Verification items for the finished model (mm, model axes). A direction names the side the tool comes from. Round coordinates to 2 decimals unless told otherwise and drop trailing zeros. Loops run counter-clockwise (first coordinate to the right, second up) from the corner with the lowest first, then second, coordinate; pieces in that order, holes last. Notation, with made-up numbers: (0.5, 0.5) - (30.5, 0.5) arc R21 cw to (30.5, 6.5) - close; hole circle Ø11 at (63, 69). An arc over 180 degrees is marked (long way). Use CSV: the item, a comma, the result in double quotes.
Autodesk Inventor part; units mm, degrees
ref_plane "YZ Plane" through (0, 0, 0) normal (1, 0, 0) x (0, 1, 0)
ref_plane "XZ Plane" through (0, 0, 0) normal (0, 1, 0) x (-1, 0, 0)
ref_plane "XY Plane" through (0, 0, 0) normal (0, 0, 1) x (1, 0, 0)
sketch "Sketch1" plane through (0, 0, 0) normal (0, 0, 1) x (1, 0, 0)
  line L0 (-35, 0) -> (0, 0)
  line L1 (0, 0) -> (0, 10)
  line L2 (0, 10) -> (-35, 10)
  line L3 (-35, 10) -> (-35, 0)
  dimension "d0" = 35
  dimension "d1" = 10
extrude "Extrusion1" add sketch "Sketch1" along normal blind 30
sketch "Sketch2" plane through (-35, 10, 0) normal (0, 1, 0) x (1, 0, 0)
  line L0 (35, -30) -> (0, -30) construction
  line L1 (17.5, -30) -> (17.5, 0) construction
  line L2 (0, 0) -> (35, 0) construction
  circle A0 centre (17.5, -15) radius 11.25
  point P0 (30, -30)
  point P1 (5, -30)
  point P2 (5, 0)
  point P3 (30, 0)
  dimension "d5" = 22.5
extrude "Extrusion2" cut sketch "Sketch2" against normal blind 7.5
sketch "Sketch3" plane through (0, 0, 0) normal (0, 0, -1) x (-1, 0, 0)
  line L0 (0, 10) -> (35, 10) construction
  line L1 (17.5, 10) -> (17.5, 0) construction
  line L2 (30, 0) -> (5, 0) construction
  circle A0 centre (4, 5) radius 1.65
  circle A1 centre (31, 5) radius 1.65
  line L3 (0, 0) -> (0, 10)
  line L4 (35, 10) -> (35, 0)
  point P0 (5, 10)
  point P1 (30, 10)
  point P2 (17.5, 5)
  point P3 (0, 5)
  point P4 (35, 5)
  dimension "d8" = 3.3
  dimension "d9" = 4
  dimension "d10" = 4
extrude "Extrusion3" cut sketch "Sketch3" against normal through all
fillet "Fillet2" radius 2 2 edges at (-35, 0, 15) (0, 0, 15)
properties part number "servo_pressfit_plate"
1) Cross-section at B-B, the plane y = 8. Record the cut outline in (x, z), then the cut area to 3 significant figures.
Returned:
outline,"(-35, 0) - (0, 0) - (0, 30) - (-35, 30) - close; hole circle Ø22.5 at (-17.5, 15)"
area,"652 mm²"
2) Access from +Z, -Z, +X, -X, +Y, -Y to the whole of each face (thin tool, end or side, straight path). Record for faces 4 (the face through (-6, 10, 15)), 5 (the face through (-18, 2.5, 15)).
Returned:
face 4,"+Z, -Z, +X, -X, +Y"
face 5,"+Y"
3) Cross-section at D-D, the plane x = -17.5. Record the cut outline in (y, z), then the cut area to 3 significant figures.
Returned:
outline,"(0, 0) - (10, 0) - (10, 3.75) - (2.5, 3.75) - (2.5, 26.25) - (10, 26.25) - (10, 30) - (0, 30) - close"
area,"131 mm²"
4) Cross-section at C-C, the plane z = 15. Record the cut outline in (x, y).
Returned:
outline,"(-35, 2) arc R2 ccw to (-33, 0) - (-2, 0) arc R2 ccw to (0, 2) - (0, 10) - (-6.25, 10) - (-6.25, 2.5) - (-28.75, 2.5) - (-28.75, 10) - (-35, 10) - close; hole circle Ø3.3 at (-31, 5); hole circle Ø3.3 at (-4, 5)"
5) Mould release check, pull along Y, two halves, no side actions. Record for faces 1 (the face through (-18, 0, 15)), 2 (the face through (-29.69, 4, 14.79)), 3 (the face through (-18, 5, 0)): +Y half, -Y half, draft (parallel to the pull), parting line (faces both ways), or undercut.
Returned:
face 1,"-Y half"
face 2,"undercut"
face 3,"draft"
6) Thickness scan on probe 1 along Y at (x, z) = (-4, 12.5); probe 2 along X at (y, z) = (6, 15); probe 3 along X at (y, z) = (8.25, 15). Record the ranges inside material, lowest first. Write a range as [from, to].
Returned:
probe 1,"y = [0, 3.35], [6.65, 10]"
probe 2,"x = [-35, -32.31], [-29.69, -28.75], [-6.25, -5.31], [-2.69, 0]"
probe 3,"x = [-35, -28.75], [-6.25, 0]"
7) Cross-section at A-A, the plane x = -4. Record the cut outline in (y, z).
Returned:
outline,"(0, 0) - (3.35, 0) - (3.35, 30) - (0, 30) - close; (6.65, 0) - (10, 0) - (10, 30) - (6.65, 30) - close"
